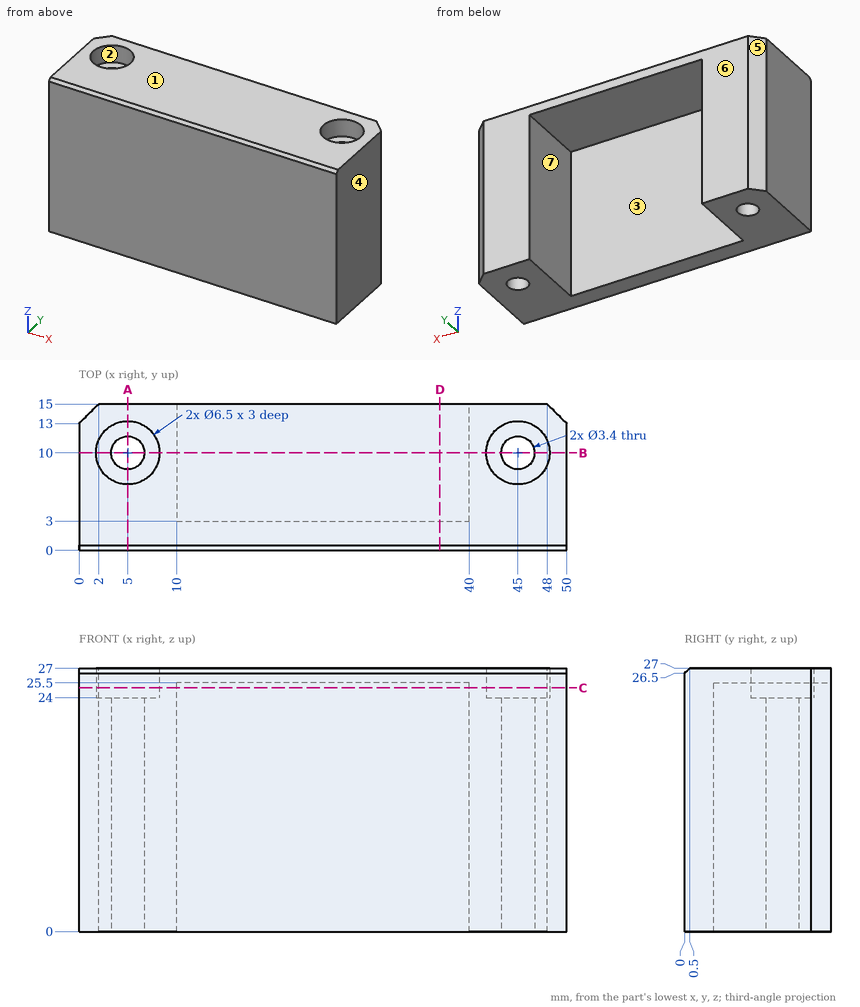
Drawing for the job (mm, zero at the part's lowest x, y, z). A direction names the side the tool comes from. Give positions to 0.01 mm unless a question says otherwise; leave off trailing zeros. Order: outer loops, then holes, each group sorted by start corner. A loop starts at its lowest first (then second) coordinate and runs counter-clockwise, first axis right, second up. Notation, with made-up numbers: M 44,17 L 49,17 A34 cw 49,50 Z; hole C -19,78 d2. An arc over 180 degrees is marked long. Put each result on its own line as item: value. Start each with the question number.
(1) Mould opens along X. For the marked faces 4, 5, 6 and 7 say: +X half, -X half, draft (parallel to the pull), parting line (faces both ways), or undercut.
(2) Saw through at C-C, the plane z = 25. Write the cut outline in (x, y), then the cut area to 3 significant figures.
(3) Saw through at A-A, the plane x = 5. Write the cut outline in (y, z).
(4) Saw through at B-B, the plane y = 10. Write the cut outline in (x, z), then the cut area to 3 significant figures.
(5) Flat gauge pins, fed straight in: pin 1 Ø3.5 at (x, y) = (32, 12) entering from -Z; pin 2 Ø6 at (x, y) = (45, 10) entering from +Z; pin 3 Ø12 at (x, z) = (20.5, 5.5) entering from +Y. Where does each tip first touch, or does it go through?
(6) Drill centre lines: line 1 along X through (y, z) = (10, 9); line 2 along X through (y, z) = (3.75, 8.25); line 3 along Y through (x, z) = (5, 14.75). Where is each one in solid material? Low to high.
(7) Which spindle directions (+Z, -Z, +X, -X, +Y, -Y) get a long thin tool onto all of the face, cutting with end or side? Do the marked faces 1, 2 and 3. Say none if no direction does.
(8) Saw through at D-D, the plane x = 37. Write the cut outline in (y, z).
Check result:
1. face 4: +X half
1. face 5: -X half
1. face 6: draft
1. face 7: undercut
2. outline: M 0,0 L 50,0 L 50,13 L 48,15 L 40,15 L 40,3 L 10,3 L 10,15 L 2,15 L 0,13 Z; hole C 5,10 d6.5; hole C 45,10 d6.5
2. area: 320 mm2
3. outline: M 0,0 L 8.3,0 L 8.3,24 L 6.75,24 L 6.75,27 L 0.5,27 L 0,26.5 Z; M 11.7,0 L 15,0 L 15,27 L 13.25,27 L 13.25,24 L 11.7,24 Z
4. outline: M 0,0 L 3.3,0 L 3.3,24 L 1.75,24 L 1.75,27 L 0,27 Z; M 6.7,0 L 10,0 L 10,25.5 L 40,25.5 L 40,0 L 43.3,0 L 43.3,24 L 41.75,24 L 41.75,27 L 8.25,27 L 8.25,24 L 6.7,24 Z; M 46.7,0 L 50,0 L 50,27 L 48.25,27 L 48.25,24 L 46.7,24 Z
4. area: 383 mm2
5. pin 1: stops at z = 25.5
5. pin 2: stops at z = 24
5. pin 3: stops at y = 3
6. line 1: x = 0 to 3.3, 6.7 to 10, 40 to 43.3, 46.7 to 50
6. line 2: x = 0 to 10, 40 to 50
6. line 3: y = 0 to 8.3, 11.7 to 15
7. face 1: +Z, +X, -X, +Y, -Y
7. face 2: +Z
7. face 3: -Z, +Y
8. outline: M 0,0 L 3,0 L 3,25.5 L 15,25.5 L 15,27 L 0.5,27 L 0,26.5 Z
